```python
from build123d import *

# Parameters (mm, degrees)
SKETCH1_R           = 85
BOSS_EXTRUDE1_DEPTH = 12
SKETCH2_R           = 75.2
CUT_EXTRUDE1_DEPTH  = 32
BOSS_EXTRUDE2_DEPTH = 16
SKETCH4_R           = 3
CUT_EXTRUDE2_DEPTH  = 44
SKETCH5_R           = 3
CUT_EXTRUDE3_DEPTH  = 44
BOSS_EXTRUDE3_DEPTH = 16
SKETCH7_R           = 3
CUT_EXTRUDE4_DEPTH  = 44
SKETCH8_R           = 3
CUT_EXTRUDE5_DEPTH  = 44
BOSS_EXTRUDE4_DEPTH = 16
SKETCH10_R          = 3
CUT_EXTRUDE6_DEPTH  = 44
SKETCH11_R          = 3
CUT_EXTRUDE7_DEPTH  = 44


with BuildPart() as part:
    # Sketch1 → Boss-Extrude1 (new body)
    with BuildSketch(Plane.XY):
        with Locations((300, 300)):
            Circle(SKETCH1_R)
    extrude(amount=BOSS_EXTRUDE1_DEPTH)

    # Sketch2 → Cut-Extrude1 (cut)
    with BuildSketch(Plane.XY.offset(12)):
        with Locations((300, 300)):
            Circle(SKETCH2_R)
    extrude(amount=-CUT_EXTRUDE1_DEPTH, mode=Mode.SUBTRACT)

    # Sketch3 → Boss-Extrude2 (add)
    with BuildSketch(Plane.XY.offset(8)):
        Polygon((360.16, 254.88), (510, 254.88), (510, 345), (360.249813278, 345), align=None)
    extrude(amount=BOSS_EXTRUDE2_DEPTH)

    # Sketch4 → Cut-Extrude2 (cut)
    with BuildSketch(Plane.XY.offset(24)):
        with Locations((480, 268)):
            Circle(SKETCH4_R)
    extrude(amount=-CUT_EXTRUDE2_DEPTH, mode=Mode.SUBTRACT)

    # Sketch5 → Cut-Extrude3 (cut)
    with BuildSketch(Plane.XY.offset(24)):
        with Locations((480, 332)):
            Circle(SKETCH5_R)
    extrude(amount=-CUT_EXTRUDE3_DEPTH, mode=Mode.SUBTRACT)

    # Sketch6 → Boss-Extrude3 (add)
    with BuildSketch(Plane.XY.offset(8)):
        Polygon((308.995066219, 374.660088292), (233.97114317, 504.365334795), (156.064945237, 459.302943285), (230.963081874, 329.815162849), align=None)
    extrude(amount=BOSS_EXTRUDE3_DEPTH)

    # Sketch7 → Cut-Extrude4 (cut)
    with BuildSketch(Plane.XY.offset(24)):
        with Locations((237.712812921, 471.884572681)):
            Circle(SKETCH7_R)
    extrude(amount=-CUT_EXTRUDE4_DEPTH, mode=Mode.SUBTRACT)

    # Sketch8 → Cut-Extrude5 (cut)
    with BuildSketch(Plane.XY.offset(24)):
        with Locations((182.287187079, 439.884572681)):
            Circle(SKETCH8_R)
    extrude(amount=-CUT_EXTRUDE5_DEPTH, mode=Mode.SUBTRACT)

    # Sketch9 → Boss-Extrude4 (add)
    with BuildSketch(Plane.XY.offset(8)):
        Polygon((230.844933781, 270.459911708), (156.02885683, 140.634665205), (234.007131599, 95.697114438), (308.697770617, 225.30469368), align=None)
    extrude(amount=BOSS_EXTRUDE4_DEPTH)

    # Sketch10 → Cut-Extrude6 (cut)
    with BuildSketch(Plane.XY.offset(24)):
        with Locations((182.287187079, 160.115427319)):
            Circle(SKETCH10_R)
    extrude(amount=-CUT_EXTRUDE6_DEPTH, mode=Mode.SUBTRACT)

    # Sketch11 → Cut-Extrude7 (cut)
    with BuildSketch(Plane.XY.offset(24)):
        with Locations((237.712812921, 128.115427319)):
            Circle(SKETCH11_R)
    extrude(amount=-CUT_EXTRUDE7_DEPTH, mode=Mode.SUBTRACT)


solid = part.part
```
The model under review builds one solid part; all positions refer to its coordinate system, in mm. A direction names the side the tool comes from. Round coordinates to 2 decimals unless told otherwise and drop trailing zeros. Write each loop counter-clockwise with the first axis right and the second up, starting at its lowest first coordinate (ties: lowest second). Pieces come first, ordered by that corner, then holes.
(1) We need section D-D on y = 364.5. Give the boundary of the cut face in (x, z), and give its area (3 significant figures).
(2) We need section B-B on x = 261. Give the boundary of the cut face in (y, z), and give its area (3 significant figures).
(3) Machinability: for faces 4 (the flat face through (340, 368, 12)), 5 (the flat face through (267, 356, 8)), 6 (the flat face through (228, 179, 8)), which of the approach directions +Z, -Z, +X, -X, +Y, -Y give a long, thin tool a straight path to every point of the face, cutting with its end or side? Answer none if there is none.
(4) Wall thickness on L1, parallel to Y at x = 480, z = 16; L2, parallel to X at y = 332, z = 14; L3, parallel to Y at x = 300, z = 6.5: over which ranges is each line inside the solid? List them lowest first.
(5) We need section C-C on z = 4.25. Give the boundary of the cut face in (x, y).
(6) Mouldability with a two-part tool opening along Y and no side actions: class faces 1 (the flat face through (223, 301, 12)), 2 (the flat face through (436, 345, 16)), 3 (the flat face through (510, 299, 16)) as +Y half, -Y half, draft (parallel to the pull), parting line (faces both ways), or undercut.
(7) Insertion check: pin 1 (8 mm diameter, centred on x = 427, z = 14.5, fed in from +Y); pin 2 (5 mm diameter, centred on x = 480, y = 268, fed in from -Z); pin 3 (10 mm diameter, centred on x = 281.5, y = 412.5, fed in from -Z); pin 4 (5 mm diameter, centred on y = 190.5, z = 7, fed in from +X). Each pin has a flat end and moves straight along its axis. Give the tip position at first contact, or say it passes through.
(8) We need section A-A on y = 300. Give the boundary of the cut face in (x, z).
Findings below:
1. outline: (210.9, 8) - (244.64, 8) - (244.64, 0) - (261.34, 0) - (261.34, 8) - (291.32, 8) - (291.32, 24) - (210.9, 24) - close; (338.66, 0) - (355.36, 0) - (355.36, 12) - (338.66, 12) - close
1. area: 1,620 mm2
2. outline: (142.54, 8) - (224.48, 8) - (224.48, 0) - (235.7, 0) - (235.7, 8) - (252.97, 8) - (252.97, 24) - (142.54, 24) - close; (347.08, 8) - (364.3, 8) - (364.3, 0) - (375.52, 0) - (375.52, 8) - (457.64, 8) - (457.64, 24) - (347.08, 24) - close
2. area: 3,720 mm2
3. face 4: +Z, +X, +Y
3. face 5: -Z
3. face 6: -Z, -X, -Y
4. L1: y = 254.88 to 265, 271 to 329, 335 to 345
4. L2: x = 229.7 to 234.76, 360.24 to 477, 483 to 510
4. L3: y = 215 to 224.8, 375.2 to 385
5. outline: circle Ø170 at (300, 300); hole circle Ø150.4 at (300, 300)
6. face 1: undercut
6. face 2: +Y half
6. face 3: draft
7. pin 1: stops at y = 345
7. pin 2: passes through
7. pin 3: stops at z = 8
7. pin 4: stops at x = 289.96
8. outline: (215, 0) - (224.8, 0) - (224.8, 12) - (215, 12) - close; (360.2, 8) - (375.2, 8) - (375.2, 0) - (385, 0) - (385, 8) - (510, 8) - (510, 24) - (360.2, 24) - close
